Build history of the part. All positions in model axes, mm. Round coordinates to 2 decimals unless told otherwise and drop trailing zeros. Loops run counter-clockwise (first coordinate to the right, second up) from the corner with the lowest first, then second, coordinate; pieces in that order, holes last. Notation, with made-up numbers: (23.5, -12) - (39.5, -12) arc R36 cw to (39.5, 22) - close; hole circle Ø11 at (20.5, 0.5). An arc over 180 degrees is marked (long way). Use one line per item in the form item = value. Start each with the question number.
Q1. Saw through at A-A (z = -95). Give the cut face in (x, y) (3 decimals), then the cut area to 3 significant figures.
Q2. Pin check, flat tips, straight feed: pin 1 (1 mm diameter, centred on x = -86.5, y = 1.5, fed in from -Z); pin 2 (3 mm diameter, centred on x = 52, z = -28, fed in from -Y); pin 3 (1.6 mm diameter, centred on x = -79.5, y = 2, fed in from -Z). Stop position of each tip, or through.
Q3. Drill centre lines: line 1 (Z direction, x = 76, y = 0.85); line 2 (X direction, y = 0.7, z = 69.85); line 3 (Z direction, x = 74, y = 1.9). Where is each one in solid material? Low to high.
Q4. Saw through at B-B (y = 0.6). Count the separate pieces of the cut face and the enclosed holes in it, then the cut area to 3 significant figures.
```python
from build123d import *

# Parameters (mm, degrees)
SKETCH1_W             = 203.2
SKETCH1_H             = 254
BOSS_EXTRUDE1_DEPTH   = 3.175
FILLET1_R             = 25.4
CUT_EXTRUDE1_DEPTH    = 25.4
FILLET2_R             = 0.762
M4X0_7_TAPPED_HOLE3_D = 3.3


with BuildPart() as part:
    # Sketch1 → Boss-Extrude1 (new body)
    with BuildSketch(Plane(origin=(0, 0, 0), x_dir=(1, 0, 0), z_dir=(0, 1, 0))):
        Rectangle(SKETCH1_W, SKETCH1_H)
    extrude(amount=BOSS_EXTRUDE1_DEPTH)

    # Fillet1
    fillet1_edges = [part.edges().sort_by_distance(p)[0] for p in [
        (101.6, 1.5875, 127),
        (-101.6, 1.5875, 127),
        (-101.6, 1.5875, -127),
        (101.6, 1.5875, -127),
    ]]
    fillet(fillet1_edges, radius=FILLET1_R)

    # Sketch2 → Cut-Extrude1 (cut)
    with BuildSketch(Plane.XZ):
        Polygon((-69.046, 73.546000013), (-69.046, 114.554000013), (-89.154, 114.554000013), (-89.154, 73.546000013), (-82.904, 73.546000013), (-82.904, 68.046000013), (-75.296, 68.046000013), (-75.296, 73.546000013), align=None)
        Polygon((75.296, 73.546000013), (69.046, 73.546000013), (69.046, 114.554000013), (89.154, 114.554000013), (89.154, 73.546000013), (82.904, 73.546000013), (82.904, 68.046000013), (75.296, 68.046000013), align=None)
        Polygon((69.046, -73.546000013), (69.046, -114.554000013), (89.154, -114.554000013), (89.154, -73.546000013), (82.904, -73.546000013), (82.904, -68.046000013), (75.296, -68.046000013), (75.296, -73.546000013), align=None)
        Polygon((-75.296, -73.546000013), (-69.046, -73.546000013), (-69.046, -114.554000013), (-89.154, -114.554000013), (-89.154, -73.546000013), (-82.904, -73.546000013), (-82.904, -68.046000013), (-75.296, -68.046000013), align=None)
    extrude(amount=-CUT_EXTRUDE1_DEPTH, mode=Mode.SUBTRACT)

    # Fillet2
    fillet2_edges = [part.edges().sort_by_distance(p)[0] for p in [
        (-69.046, 1.5875, 73.546000013),
        (-75.296, 1.5875, 73.546000013),
        (-75.296, 1.5875, 68.046000013),
        (-82.904, 1.5875, 68.046000013),
        (-82.904, 1.5875, 73.546000013),
        (-89.154, 1.5875, 73.546000013),
        (-89.154, 1.5875, 114.554000013),
        (-69.046, 1.5875, 114.554000013),
        (-82.904, 1.5875, -68.046000013),
        (-75.296, 1.5875, -68.046000013),
        (-75.296, 1.5875, -73.546000013),
        (-69.046, 1.5875, -73.546000013),
        (-69.046, 1.5875, -114.554000013),
        (-89.154, 1.5875, -114.554000013),
        (-89.154, 1.5875, -73.546000013),
        (-82.904, 1.5875, -73.546000013),
        (69.046, 1.5875, -73.546000013),
        (75.296, 1.5875, -73.546000013),
        (75.296, 1.5875, -68.046000013),
        (82.904, 1.5875, -68.046000013),
        (82.904, 1.5875, -73.546000013),
        (89.154, 1.5875, -73.546000013),
        (89.154, 1.5875, -114.554000013),
        (69.046, 1.5875, -114.554000013),
        (82.904, 1.5875, 68.046000013),
        (75.296, 1.5875, 68.046000013),
        (75.296, 1.5875, 73.546000013),
        (69.046, 1.5875, 73.546000013),
        (69.046, 1.5875, 114.554000013),
        (89.154, 1.5875, 114.554000013),
        (89.154, 1.5875, 73.546000013),
        (82.904, 1.5875, 73.546000013),
    ]]
    fillet(fillet2_edges, radius=FILLET2_R)

    # M4x0.7 Tapped Hole3 (through all)
    with Locations(Plane(origin=(0, 3.175, 0), x_dir=(1, 0, 0), z_dir=(0, 1, 0))):
        with Locations((-84.2, -69.850000013), (-74, -118.250000013), (74, -118.250000013), (84.2, -69.850000013), (84.2, 69.850000013), (74, 118.250000013), (-74, 118.250000013), (-84.2, 69.850000013)):
            Hole(M4X0_7_TAPPED_HOLE3_D / 2)


solid = part.part
```
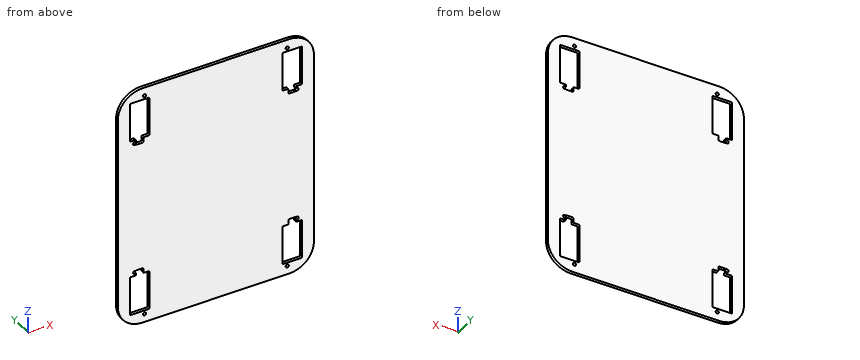
Report:
q1.outline = (-101.6, 0) - (-89.154, 0) - (-89.154, 3.175) - (-101.6, 3.175) - close; (-69.046, 0) - (69.046, 0) - (69.046, 3.175) - (-69.046, 3.175) - close; (89.154, 0) - (101.6, 0) - (101.6, 3.175) - (89.154, 3.175) - close
q1.area = 517 mm²
q2.pin_1 = -125.03
q2.pin_2 = 0
q2.pin_3 = -126.88
q3.line_1 = -127 to -114.55, -68.05 to 68.05, 114.55 to 127
q3.line_2 = -101.6 to -85.85, -75.3 to 75.3, 85.85 to 101.6
q3.line_3 = -127 to -119.9, -116.6 to -114.55, -73.55 to 73.55, 114.55 to 116.6, 119.9 to 127
q4.separate_pieces = 1
q4.enclosed_holes = 8
q4.area = 47,500 mm²
